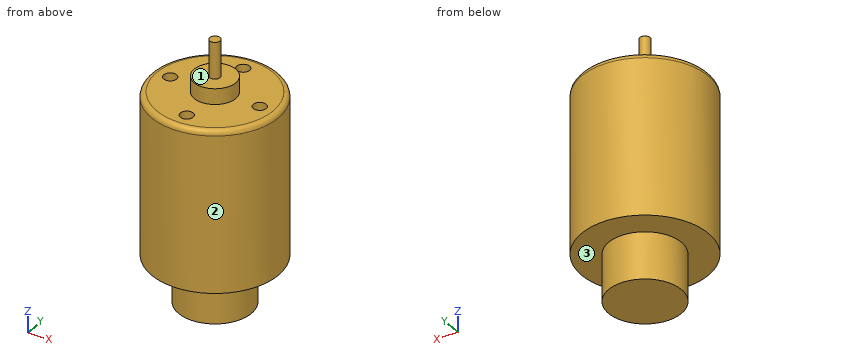
from build123d import *

# Parameters (mm, degrees)
ESBO_O1_R                                   = 12.2
RESSALTO_EXTRUS_O1_DEPTH                    = 31
BROCA_DE_ROSQUEAR_PARA_TARRAXA_DE_M31_D     = 2.5
BROCA_DE_ROSQUEAR_PARA_TARRAXA_DE_M31_DEPTH = 3
BROCA_DE_ROSQUEAR_PARA_TARRAXA_DE_M31_TIP   = 0.751075774
ESBO_O5_R                                   = 4
RESSALTO_EXTRUS_O2_DEPTH                    = 3
ESBO_O6_R                                   = 1
RESSALTO_EXTRUS_O3_DEPTH                    = 7
ESBO_O7_R                                   = 7
RESSALTO_EXTRUS_O4_DEPTH                    = 9
FILETE1_R                                   = 1


with BuildPart() as part:
    # Esboço1 → Ressalto-extrusão1 (new body)
    with BuildSketch(Plane.XY):
        Circle(ESBO_O1_R)
    extrude(amount=RESSALTO_EXTRUS_O1_DEPTH)

    # Broca de rosquear para tarraxa de M31
    with Locations(Plane(origin=(-8.6, 0, 31), x_dir=(1, 0, 0), z_dir=(0, 0, 1))):
        with Locations((0, 0), (8.6, 8.6), (17.2, 0), (8.6, -8.6)):
            Hole(BROCA_DE_ROSQUEAR_PARA_TARRAXA_DE_M31_D / 2, depth=BROCA_DE_ROSQUEAR_PARA_TARRAXA_DE_M31_DEPTH)
            with Locations((0, 0, -(BROCA_DE_ROSQUEAR_PARA_TARRAXA_DE_M31_DEPTH + BROCA_DE_ROSQUEAR_PARA_TARRAXA_DE_M31_TIP / 2))):  # 118° drill point
                Cone(0, BROCA_DE_ROSQUEAR_PARA_TARRAXA_DE_M31_D / 2, BROCA_DE_ROSQUEAR_PARA_TARRAXA_DE_M31_TIP, mode=Mode.SUBTRACT)

    # Esboço5 → Ressalto-extrusão2 (add)
    with BuildSketch(Plane.XY.offset(31)):
        Circle(ESBO_O5_R)
    extrude(amount=RESSALTO_EXTRUS_O2_DEPTH)

    # Esboço6 → Ressalto-extrusão3 (add)
    with BuildSketch(Plane.XY.offset(34)):
        Circle(ESBO_O6_R)
    extrude(amount=RESSALTO_EXTRUS_O3_DEPTH)

    # Esboço7 → Ressalto-extrusão4 (add)
    with BuildSketch(Plane(origin=(0, 0, 0), x_dir=(-1, 0, 0), z_dir=(0, 0, -1))):
        Circle(ESBO_O7_R)
    extrude(amount=RESSALTO_EXTRUS_O4_DEPTH)

    # Filete1
    filete1_edges = [part.edges().sort_by_distance(p)[0] for p in [
        (-12.2, 0, 31),
    ]]
    fillet(filete1_edges, radius=FILETE1_R)


solid = part.part
The listing builds one solid part. Answer for the finished solid, in the listing's coordinates (mm). Face numbers are marked on the shaded views. A direction names the side the tool comes from. Coordinates: 2 decimals unless noted, no trailing zeros. Write each loop counter-clockwise with the first axis right and the second up, starting at its lowest first coordinate (ties: lowest second). Pieces come first, ordered by that corner, then holes. Notation, with made-up numbers: (-26, 46) - (-8, 46) arc R10 cw to (-8, 60) - close; hole circle Ø5 at (27, 39). An arc over 180 degrees is marked (long way). Return JSON: item names as keys, results as strings.
1. The part is cut by section A-A on z = 29.5. Determine the outline of the cut face in (x, y).
Final values:
{"outline": "circle Ø24.4 at (0, 0); hole circle Ø2.5 at (-8.6, 0); hole circle Ø2.5 at (0, -8.6); hole circle Ø2.5 at (0, 8.6); hole circle Ø2.5 at (8.6, 0)"}
2. The part is cut by section C-C on z = 24. Determine the outline of the cut face in (x, y).
Final values:
{"outline": "circle Ø24.4 at (0, 0)"}
3. Each of these flat-tipped pins is pushed along its axis until it touches: pin 1 Ø1.5 at (x, y) = (0, -8.6) entering from +Z; pin 2 Ø8 at (y, z) = (-7.5, 10) entering from +X; pin 3 Ø6 at (x, z) = (8.5, 14) entering from -Y. Where does it stop, or does it pass through?
Final values:
{"pin 1": "z = 27.7", "pin 2": "x = 11.69", "pin 3": "y = -10.89"}
4. Consider line 1 along Y through (x, z) = (0, 30); line 2 along Z through (x, y) = (3.75, -4.75); line 3 along Z through (x, y) = (-3.75, -9). Determine where each line is inside the solid, lowest interval first.
Final values:
{"line 1": "-12.2 to -9.85, -7.35 to 7.35, 9.85 to 12.2", "line 2": "-9 to 31", "line 3": "0 to 31"}
5. The part is cut by section B-B on z = 34.5. Determine the outline of the cut face in (x, y), then the cut area to 3 significant figures.
Final values:
{"outline": "circle Ø2 at (0, 0)", "area": "3.14 mm^2"}
6. Which of the six approach directions +Z, -Z, +X, -X, +Y, -Y give full straight-line access (tool end or side, diameter ignored) to the marked faces 1, 2 and 3?
Final values:
{"face 1": "+Z", "face 2": "+Z, -Z", "face 3": "-Z"}
